Geometry: final body of the model. Coordinates: model frame, mm. Give positions to 0.01 mm unless a question says otherwise; leave off trailing zeros. Write each loop counter-clockwise with the first axis right and the second up, starting at its lowest first coordinate (ties: lowest second). Pieces come first, ordered by that corner, then holes. Notation, with made-up numbers: M 10,39.25 L 17,39.25 A22 cw 17,45.25 Z; hole C -36.75,41 d11. An arc over 180 degrees is marked long. Use a Markdown table: item, result. Add a question column.
(1) Cut plane B-B (y = -20). State how many separate pieces and enclosed holes the cut face has, plus the area to 3 significant figures.
(2) Cut plane A-A (y = 0). Output: boundary loops of the cut face in (x, z), plus the area to 3 significant figures.
(3) Draft query along X for faces 1 (the conical face through (-34.132, -18.3, 4.084)), 2 (the flat face through (-1, 6, 6.35)), 3 (the conical face through (29.368, -18.3, 4.084)), 4 (the cylindrical face through (36.29, 23.49, 3.22)). Return one class per face: released by +X, released by -X, zero draft, split by the parting line, or undercut.
(4) Pin query (flat end, axial travel): pin 1 Ø6 at (x, y) = (-31.75, 19.05) entering from +Z; pin 2 Ø5.5 at (x, y) = (31.75, 19.05) entering from +Z. Return the tip coordinate at first contact, or that it passes through.
(5) Material intervals for L1, parallel to X at y = 19.05, z = 2.9; L2, parallel to Y at x = -31.75, z = 2.4; L3, parallel to Y at x = -32.5, z = 4.25, sorted ascending.
```python
from build123d import *

# Parameters (mm, degrees)
F1_W           = 76.2
F1_H           = 50.8
F2_DEPTH       = 6.35
F3_R           = 6.35
F5_D           = 4.7625
F5_CSINK_D     = 9.525
F5_CSINK_ANGLE = 90
F6_D           = 5.1054


with BuildPart() as f2:
    # F1 (on Top) → F2 (new body)
    with BuildSketch(Plane.XY):
        Rectangle(F1_W, F1_H)
    extrude(amount=F2_DEPTH)

    # F3
    f3_edges = [f2.edges().sort_by_distance(p)[0] for p in [
        (-38.1, -25.4, 3.175),
        (38.1, -25.4, 3.175),
        (38.1, 25.4, 3.175),
        (-38.1, 25.4, 3.175),
    ]]
    fillet(f3_edges, radius=F3_R)

    # F5 (through all)
    with Locations(Plane.XY.offset(6.35)):
        with Locations((-31.75, 19.05), (-31.75, -19.05), (31.75, -19.05), (31.75, 19.05)):
            CounterSinkHole(F5_D / 2, F5_CSINK_D / 2, counter_sink_angle=F5_CSINK_ANGLE)

    # F6 (through all)
    with Locations(Plane(origin=(0, 0, 0), x_dir=(1, 0, 0), z_dir=(0, 0, -1))):
        with Locations((0, 0)):
            Hole(F6_D / 2)


solid = f2.part
```
Answer list:
| question | item | result |
|---|---|---|
| 1 | separate pieces | 3 |
| 1 | enclosed holes | 0 |
| 1 | area | 416 mm² |
| 2 | outline | M -38.1,0 L -2.55,0 L -2.55,6.35 L -38.1,6.35 Z; M 2.55,0 L 38.1,0 L 38.1,6.35 L 2.55,6.35 Z |
| 2 | area | 451 mm² |
| 3 | face 1 | undercut |
| 3 | face 2 | zero draft |
| 3 | face 3 | undercut |
| 3 | face 4 | released by +X |
| 4 | pin 1 | z = 4.59 |
| 4 | pin 2 | z = 4.34 |
| 5 | L1 | -38.1 to -34.13, -29.37 to 29.37, 34.13 to 38.1 |
| 5 | L2 | -25.4 to -21.43, -16.67 to 16.67, 21.43 to 25.4 |
| 5 | L3 | -25.36 to -21.6, -16.5 to 16.5, 21.6 to 25.36 |
